Could you check a few things on this model? Use its own coordinates, in mm. A direction names the side the tool comes from. Coordinates: 2 decimals unless noted, no trailing zeros. Loops run counter-clockwise (first coordinate to the right, second up) from the corner with the lowest first, then second, coordinate; pieces in that order, holes last. Notation, with made-up numbers: M 30.5,-35 L 53.5,-35 A12 ccw 53.5,-27 Z; hole C 51,1.5 d11. An arc over 180 degrees is marked long. Use one line per item in the form item = value. Start each with the question number.
Autodesk Inventor part; units mm, degrees
ref_plane "YZ Plane" through (0, 0, 0) normal (1, 0, 0) x (0, 1, 0)
ref_plane "XZ Plane" through (0, 0, 0) normal (0, 1, 0) x (-1, 0, 0)
ref_plane "XY Plane" through (0, 0, 0) normal (0, 0, 1) x (1, 0, 0)
sketch "Skizze1" plane through (0, 0, 0) normal (0, 0, 1) x (1, 0, 0)
  circle A0 centre (4.9, 19.6) radius 0.455
  circle A1 centre (4.9, 19.6) radius 0.7
  line L0 (6.3, 18.375) -> (6.3, 19.6)
  line L1 (0, 23.5) -> (7, 23.5)
  line L2 (7, 23.5) -> (7, 22.25)
  line L3 (7, 22.25) -> (1.75, 22.25)
  line L4 (0, 0) -> (9.5856, 0)
  line L5 (0, 23.5) -> (0, 19.6)
  line L6 (0, 19.6) -> (1.75, 19.25)
  line L7 (1.75, 19.25) -> (4.9, 17.5)
  line L8 (4.9, 17.5) -> (6.3, 18.375)
  line L9 (4.9, 17.5) -> (0, 17.5) construction
  line L10 (0, 18) -> (0, -3)
  line L11 (-1.9171, 0) -> (11.5027, 0)
  line L12 (4.2, 19.6) -> (1.75, 20.09)
  line L13 (1.75, 20.09) -> (1.75, 22.25)
  line L14 (6.3, 19.6) -> (5.6, 19.6)
  dimension "d0" = 47
  dimension "d1" = 36.75
  dimension "d2" = 1.25
  dimension "d3" = 0.91
  dimension "d4" = 1.4
  dimension "d5" = 35
  dimension "d6" = 38.5
  dimension "d7" = 39.2
  dimension "d8" = 4.9
  dimension "d9" = 6.3
  dimension "d10" = 7
  dimension "d12" = 1.75
revolve "Körper" add sketch "Skizze1" angle 360 about axis through (0, 0, 0) along (1, 0, 0) contours L14 L0 L8 L7 L6 L5 L1 L2 L3 L13 L12 A1
revolve "Feder1" add sketch "Skizze1" angle 360 about axis through (0, 0, 0) along (1, 0, 0) contours A0 | A1
fillet "Rundung1" radius 0.4 3 edges at (7, -23.5, 0) (1.75, -22.25, 0) (0, -23.5, 0)
equation "\"d0\" = SD2"
equation "\"d1\" = ABDM"
equation "\"d3\" = SPDI"
equation "\"d4\" = SPDA"
equation "\"d5\" = NND"
equation "\"d6\" = TKDM"
equation "\"d7\" = HLDM"
equation "\"d8\" = SPDST"
equation "\"d9\" = SDI"
equation "\"d10\" = SWDT"
equation "\"d12\" = SD"
equation "\"d11\" = RR"
equation "\"SD2\" = 47"
equation "\"SWDT\" = 7"
equation "\"RR\" = 0.4"
equation "\"SD\" = 1.75"
equation "\"NND\" = 35"
equation "\"SPDA\" = 1.4"
equation "\"SPDI\" = 0.91"
equation "\"TKDM\" = 38.5"
equation "\"HLDM\" = 39.2"
equation "\"ABDM\" = 36.75"
equation "\"SDI\" = 6.3"
equation "\"SPDST\" = 4.9"
equation "\"LAB\" = 0.35"
properties part number "DIN 3760 - A - 35 x 47 x 7 - NBR" material "Gummi"
Item 1: Please list where these lines run through material, in increasing order: line 1 along Z through (x, y) = (4.45, 0); line 2 along Z through (x, y) = (5.75, -3.5); line 3 along Z through (x, y) = (6.5, 13.5).
Item 2: I want a section at C-C (x = 3.5). Write out the boundary of the cut face in (y, z), plus the area to 3 significant figures.
Item 3: Thinking about a two-plate mould opening in Z: for faces 3 (the cylindrical face through (3.5, 22.4, 7.1)), 4 (the flat face through (7, -12, 19)), 5 (the conical face through (4.047, 9.058, 17.416)), which applies, pulls with the +Z half, pulls with the -Z half, needs draft (parallel to the pull), parting line crosses it, or undercut?
Item 4: I'm going to push flat-ended pins straight in: P1, Ø2, axis at x = 2.5, y = 5.5, coming from the -Z side; P2, Ø2, axis at y = 4, z = 14, coming from the -X side; P3, Ø3, axis at x = 1.5, y = 13, coming from the -Z side; P4, Ø1.5, axis at x = 5, y = -8.5, coming from the +Z side. Where does each tip first touch, or does it pass through?
Item 5: For faces 1 (the conical face through (4.703, -17.592, -0.774)), 2 (the cylindrical face through (4.541, -16.399, -15.038)), which set-ups out of +Z, -Z, +X, -X, +Y, -Y let a thin tool reach every point of the face, with its end or its side?
Worked answers:
q1.line_1 = -23.5 to -22.25, -20.14 to -17.75, 17.75 to 20.14, 22.25 to 23.5
q1.line_2 = -23.24 to -21.97, -19.28 to -17.69, 17.69 to 19.28, 21.97 to 23.24
q1.line_3 = -19.24 to -17.69, 17.69 to 19.24
q2.outline = C 0,0 d47; C 0,0 d39.48; hole C 0,0 d44.5; hole C 0,0 d36.56
q2.area = 354 mm²
q3.face_3 = parting line crosses it
q3.face_4 = needs draft
q3.face_5 = undercut
q4.P1 = -23.07
q4.P2 = through
q4.P3 = -20.49
q4.P4 = 22.19
q5.face_1 = -X
q5.face_2 = +X
